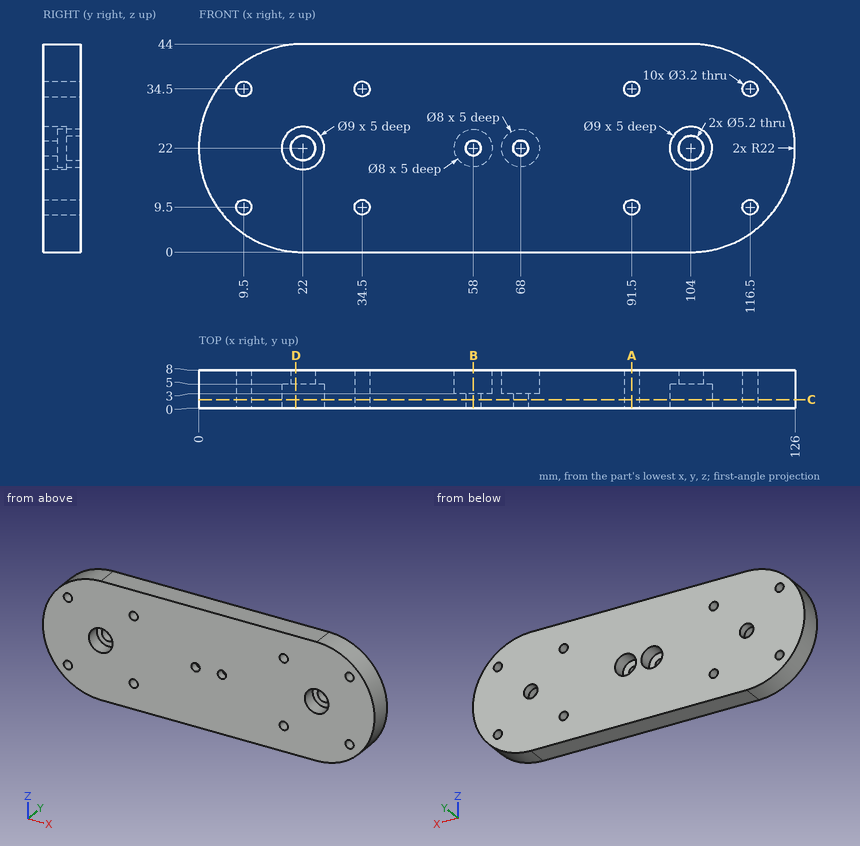
Answer from the drawing. Dimensions are ordinates in mm from the lowest x, y and z of the part. Round coordinates to 2 decimals unless told otherwise and drop trailing zeros. Order: outer loops, then holes, each group sorted by start corner. A loop starts at its lowest first (then second) coordinate and runs counter-clockwise, first axis right, second up. Notation, with made-up numbers: (-11.5, 27.5) - (-0.5, 27.5) arc R30 ccw to (-0.5, 63.5) - close; hole circle Ø4 at (74.25, 29). An arc over 180 degrees is marked (long way). Put each result on its own line as item: value. Start each with the question number.
(1) Straight lines are drawn through the part: probe 1 along X at (y, z) = (3.4, 22); probe 2 along X at (y, z) = (1, 22); probe 3 along X at (y, z) = (2.75, 26). For each, find the intervals that lie inside material, in ascending order. Write a range as from..to.
(2) Find section A-A (x = 91.5). Give the vertices of the cut face in (y, z).
(3) Find section C-C (y = 1.75). State how many separate pieces and enclosed holes the cut face has, plus the area to 3 significant figures.
(4) Find section B-B (x = 58). Give the vertices of the cut face in (y, z), plus the area to 3 significant figures.
(5) Find section D-D (x = 20.5). Give the vertices of the cut face in (y, z).
(6) Given P1, Ø5.5, axis at x = 104, z = 22, coming from the -Y side; P2, Ø6.5, axis at x = 58.5, z = 21.5, coming from the +Y side; P3, Ø1.5, axis at y = 7, z = 30.5, coming from the +X side, each flat-ended and moving along its own axis, determine where each tip first touches the part or whether it passes through.
Reply:
1. probe 1: 0..17.5, 26.5..54, 62..64, 72..99.5, 108.5..126
1. probe 2: 0..17.5, 26.5..56.4, 59.6..66.4, 69.6..99.5, 108.5..126
1. probe 3: 0.37..19.94, 24.06..101.94, 106.06..125.63
2. outline: (0, 0) - (8, 0) - (8, 7.9) - (0, 7.9) - close; (0, 11.1) - (8, 11.1) - (8, 32.9) - (0, 32.9) - close; (0, 36.1) - (8, 36.1) - (8, 44) - (0, 44) - close
3. separate pieces: 1
3. enclosed holes: 12
3. area: 4,920 mm^2
4. outline: (0, 0) - (8, 0) - (8, 18) - (3, 18) - (3, 20.4) - (0, 20.4) - close; (0, 23.6) - (3, 23.6) - (3, 26) - (8, 26) - (8, 44) - (0, 44) - close
4. area: 302 mm^2
5. outline: (0, 0.05) - (8, 0.05) - (8, 19.88) - (5, 19.88) - (5, 17.76) - (0, 17.76) - close; (0, 26.24) - (5, 26.24) - (5, 24.12) - (8, 24.12) - (8, 43.95) - (0, 43.95) - close
6. P1: y = 5
6. P2: y = 3
6. P3: x = 124.59
